Design review of the part built by this model. Coordinates are the model's own, in mm. A direction names the side the tool comes from. Coordinates: 2 decimals unless noted, no trailing zeros. Write each loop counter-clockwise with the first axis right and the second up, starting at its lowest first coordinate (ties: lowest second). Pieces come first, ordered by that corner, then holes.
Q1. Take a section at B-B (z = 0). Give the boundary of the cut face in (x, y), and give its area (3 significant figures).
Q2. Mouldability with a two-part tool opening along X and no side actions: class faces 1 (the cylindrical face through (0.888, 14.696, 0.323)), 2 (the flat face through (-7, -6, 0)), 3 (the flat face through (10, -5, 0)), 4 (the flat face through (1, -13, -15.7)) as pulls with the +X half, pulls with the -X half, needs draft (parallel to the pull), parting line crosses it, or undercut.
Q3. For probe 1 along Y at (x, z) = (-1.25, 0); probe 2 along X at (y, z) = (-9.5, 0); probe 3 along Z at (x, y) = (-3.5, -20.5), list the stretches that pass through material, from the lowest coordinate up.
Q4. Insertion check: pin 1 (5 mm diameter, centred on x = 1, z = -5, fed in from +Y); pin 2 (5 mm diameter, centred on x = 6, y = 4, fed in from -Z); pin 3 (13 mm diameter, centred on y = 0, z = 0, fed in from -X); pin 4 (2 mm diameter, centred on x = -0.5, z = 12, fed in from -Y). Each pin has a flat end and moves straight along its axis. Give the tip position at first contact, or say it passes through.
Q5. Machinability: for faces 5 (the cylindrical face through (0.89, 4.88, 1.08)), 6 (the flat face through (1, -14, 15.7)), 7 (the flat face through (1, -14, 14.7)), which of the approach directions +Z, -Z, +X, -X, +Y, -Y give a long, thin tool a straight path to every point of the face, cutting with its end or side? Answer none if there is none.
Q6. Take a section at C-C (y = 2). Give the boundary of the cut face in (x, z), and give its area (3 significant figures).
Q7. Take a section at D-D (y = -11). Give the boundary of the cut face in (x, z), and give its area (3 significant figures).
Q8. Take a section at A-A (x = 6.25). Give the boundary of the cut face in (y, z), and give its area (3 significant figures).
Autodesk Inventor part; units mm, degrees
ref_plane "Arbeitsebene1" through (0, 0, 0) normal (1, 0, 0) x (0, 0, -1)
ref_plane "YZ Plane" through (0, 0, 0) normal (1, 0, 0) x (0, 1, 0)
ref_plane "XZ Plane" through (0, 0, 0) normal (0, 1, 0) x (-1, 0, 0)
ref_plane "Arbeitsebene1" through (0, 0, 0) normal (1, 0, 0) x (0, 0, -1)
sketch "Skizze1" plane through (0, 0, 0) normal (1, 0, 0) x (0, 0, -1)
  arc A0 (15.7, 0) -> (-15.7, 0) centre (0, 0) ccw
  line L0 (15.7, 0) -> (15.7, -26.8)
  line L1 (15.7, -26.8) -> (-15.7, -26.8)
  line L2 (-15.7, -26.8) -> (-15.7, 0)
  circle A1 centre (0, 0) radius 4
  point P0 (0, 15.7)
  dimension "d0" = 31.4
  dimension "d1" = 42.5
  dimension "d2" = 8
extrude "Extrusion1" add sketch "Skizze1" along normal blind 10 and the other way blind 8
shell "Wandung1" thickness 1 removed faces 1 at (-2, -26.8, -5.2333)
properties part number "EncoderEnclosure"
Response:
1. outline: (-8, -26.8) - (-7, -26.8) - (-7, -5) - (9, -5) - (9, -26.8) - (10, -26.8) - (10, -4) - (-8, -4) - close; (-8, 4) - (10, 4) - (10, 15.7) - (-8, 15.7) - close; hole (-7, 5) - (9, 5) - (9, 14.7) - (-7, 14.7) - close
1. area: 117 mm2
2. face 1: undercut
2. face 2: undercut
2. face 3: pulls with the +X half
2. face 4: needs draft
3. probe 1: y = -5 to -4, 4 to 5, 14.7 to 15.7
3. probe 2: x = -8 to -7, 9 to 10
3. probe 3: z = -15.7 to -14.7, 14.7 to 15.7
4. pin 1: stops at y = 15.5
4. pin 2: stops at z = -15.63
4. pin 3: stops at x = -8
4. pin 4: stops at y = 6.86
5. face 5: none
5. face 6: +Z, +X, -X, +Y, -Y
5. face 7: -Y
6. outline: (-8, -15.57) - (10, -15.57) - (10, -3.46) - (-8, -3.46) - close; (-8, 3.46) - (10, 3.46) - (10, 15.57) - (-8, 15.57) - close; hole (-7, -14.56) - (9, -14.56) - (9, -4.58) - (-7, -4.58) - close; hole (-7, 4.58) - (9, 4.58) - (9, 14.56) - (-7, 14.56) - close
6. area: 117 mm2
7. outline: (-8, -15.7) - (10, -15.7) - (10, 15.7) - (-8, 15.7) - close; hole (-7, -14.7) - (9, -14.7) - (9, 14.7) - (-7, 14.7) - close
7. area: 94.8 mm2
8. outline: (-26.8, -15.7) - (0, -15.7) arc R15.7 ccw to (0, 15.7) - (-26.8, 15.7) - (-26.8, 14.7) - (0, 14.7) arc R14.7 cw to (0, -14.7) - (-26.8, -14.7) - close; circle Ø10 at (0, 0); hole circle Ø8 at (0, 0)
8. area: 130 mm2
